Study the drawing (mm; zero at the part's minimum x, y, z) and answer. Coordinates: 2 decimals unless noted, no trailing zeros. Loops run counter-clockwise (first coordinate to the right, second up) from the corner with the lowest first, then second, coordinate; pieces in that order, holes last. Notation, with made-up numbers: (-30, 74.5) -> (16, 74.5) arc R20 cw to (16, 93.5) -> close; hole circle Ø3 at (-7, -16.75). An arc over 180 degrees is marked (long way). Answer as CSV lines item,"result".
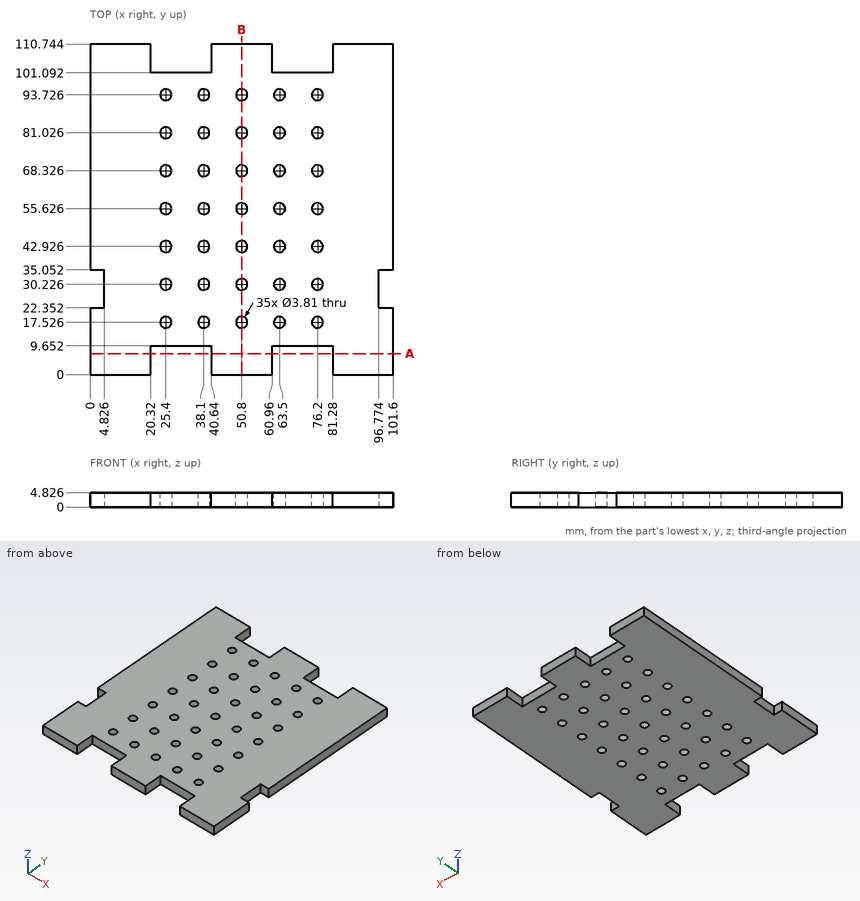
Q1. Given pin 1 Ø2.5 at (x, y) = (50.8, 55.626) entering from +Z; pin 2 Ø1.4 at (x, z) = (68, 3) entering from -Y; pin 3 Ø1 at (y, z) = (28.5, 3.5) entering from -X, each flat-ended and moving along its own axis, determine where each tip first touches the part or whether it passes through.
Results:
pin 1,"passes through"
pin 2,"stops at y = 9.65"
pin 3,"stops at x = 4.83"
Q2. A cutting plane is placed at B-B, the plane x = 50.8. Give the number of separate pieces and of enclosed holes in the cut face, and give its area (3 significant figures).
Results:
separate pieces,"8"
enclosed holes,"0"
area,"406 mm²"
Q3. A cutting plane is placed at A-A, the plane y = 7. Write down the section's boundary in (x, z).
Results:
outline,"(0, 0) -> (20.32, 0) -> (20.32, 4.83) -> (0, 4.83) -> close; (40.64, 0) -> (60.96, 0) -> (60.96, 4.83) -> (40.64, 4.83) -> close; (81.28, 0) -> (101.6, 0) -> (101.6, 4.83) -> (81.28, 4.83) -> close"
Q4. Find the intervals of material crossed by probe 1 along X at (y, z) = (7.5, 2.05); probe 2 along X at (y, z) = (30.5, 1.5); probe 3 along X at (y, z) = (68.5, 3.25), in increasing order. Write a range as [from, to].
Results:
probe 1,"x = [0, 20.32], [40.64, 60.96], [81.28, 101.6]"
probe 2,"x = [4.83, 23.51], [27.29, 36.21], [39.99, 48.91], [52.69, 61.61], [65.39, 74.31], [78.09, 96.77]"
probe 3,"x = [0, 23.5], [27.3, 36.2], [40, 48.9], [52.7, 61.6], [65.4, 74.3], [78.1, 101.6]"
